Work out the finished part from the listing and answer in its coordinate system (mm). A direction names the side the tool comes from. Give positions to 0.01 mm unless a question says otherwise; leave off trailing zeros. Order: outer loops, then holes, each group sorted by start corner. A loop starts at its lowest first (then second) coordinate and runs counter-clockwise, first axis right, second up.
```python
from build123d import *

# Parameters (mm, degrees)
BOSS_EXTRUDE1_DEPTH      = 914.4
BOSS_EXTRUDE1_DEPTH_BACK = 914.4
FILLET1_R                = 2.54


with BuildPart() as part:
    # Sketch4 → Boss-Extrude1 (new body, two sides)
    with BuildSketch(Plane.XY) as boss_extrude1_sk:
        with BuildLine():
            Line((-31.75, -29.21), (-31.75, 38.1))
            Line((-31.75, 38.1), (-38.1, 38.1))
            Line((-38.1, 38.1), (-38.1, -38.1))
            Line((-38.1, -38.1), (38.1, -38.1))
            Line((38.1, -38.1), (38.1, -31.75))
            Line((38.1, -31.75), (-29.21, -31.75))
            ThreePointArc((-29.21, -31.75), (-31.006051224, -31.006051224), (-31.75, -29.21))
        make_face()
    extrude(amount=BOSS_EXTRUDE1_DEPTH)
    extrude(boss_extrude1_sk.sketch, amount=-BOSS_EXTRUDE1_DEPTH_BACK)

    # Fillet1
    fillet1_edges = [part.edges().sort_by_distance(p)[0] for p in [
        (-31.75, 38.1, 0),
        (38.1, -31.75, 0),
        (38.1, -38.1, 0),
        (-38.1, -38.1, 0),
        (-38.1, 38.1, 0),
    ]]
    fillet(fillet1_edges, radius=FILLET1_R)


solid = part.part
```
1. Straight lines are drawn through the part: probe 1 along X at (y, z) = (19, -252); probe 2 along X at (y, z) = (-31.5, -430). For each, find the intervals that lie inside material, in ascending order.
Findings below:
probe 1: x = -38.1 to -31.75
probe 2: x = -38.1 to -30.31
2. Which of the six approach directions +Z, -Z, +X, -X, +Y, -Y give full straight-line access (tool end or side, diameter ignored) to faces 1 (the face through (-38.1, 0, 13)), 2 (the face through (-31.75, 3, 13))?
Findings below:
face 1: +Z, -Z, -X, +Y, -Y
face 2: +Z, -Z, +X, +Y
3. The part is cut by section A-A (z = 256.5). Write down the section's boundary in (x, y).
Findings below:
outline: (-38.1, -35.56) arc R2.54 ccw to (-35.56, -38.1) - (35.56, -38.1) arc R2.54 ccw to (38.1, -35.56) - (38.1, -34.29) arc R2.54 ccw to (35.56, -31.75) - (-29.21, -31.75) arc R2.54 cw to (-31.75, -29.21) - (-31.75, 35.56) arc R2.54 ccw to (-34.29, 38.1) - (-35.56, 38.1) arc R2.54 ccw to (-38.1, 35.56) - close
4. The part is cut by section B-B (y = 9.5). Write down the section's boundary in (x, z), then the cut area to 3 significant figures.
Findings below:
outline: (-38.1, -914.4) - (-31.75, -914.4) - (-31.75, 914.4) - (-38.1, 914.4) - close
area: 11,600 mm2
5. Given P1, Ø1, axis at y = -3.5, z = 412, coming from the +X side; P2, Ø10, axis at x = 2.5, z = -370.5, coming from the +Y side, each flat-ended and moving along its own axis, determine where each tip first touches the part or whether it passes through.
Findings below:
P1: stops at x = -31.75
P2: stops at y = -31.75
